Job drawing, mm, ordinate dimensions from the low corner. One solid piece. A direction names the side the tool comes from. Coordinates: 2 decimals unless noted, no trailing zeros. Write each loop counter-clockwise with the first axis right and the second up, starting at its lowest first coordinate (ties: lowest second). Pieces come first, ordered by that corner, then holes.
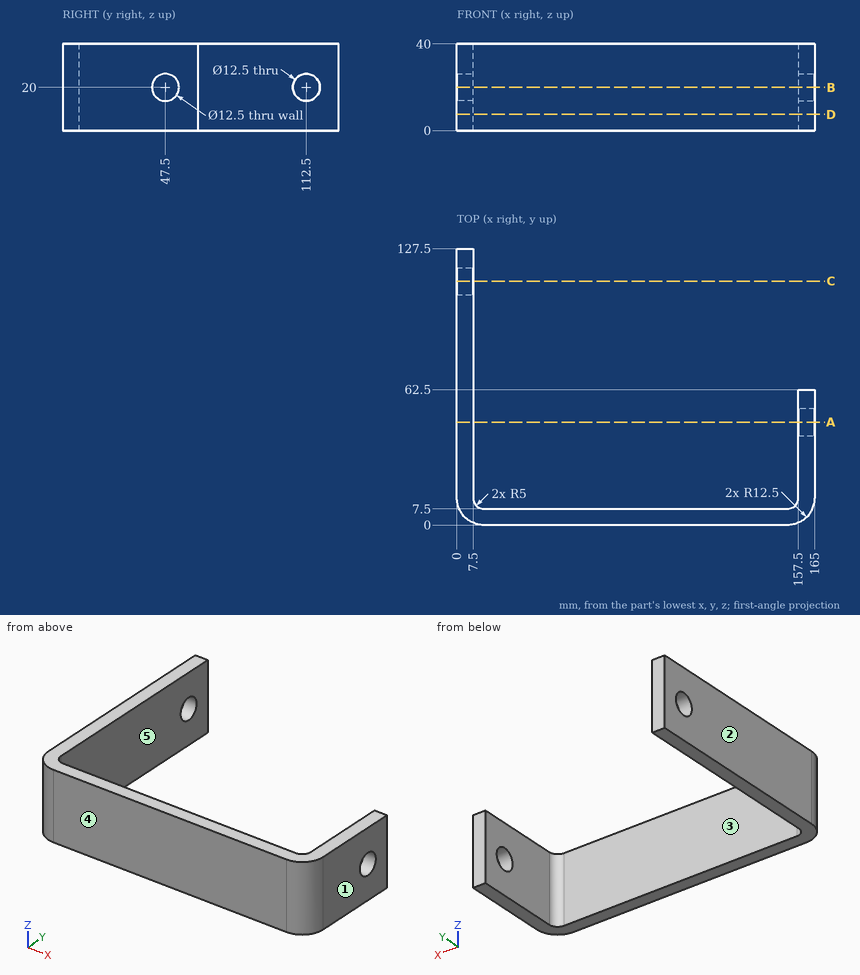
1. Flat gauge pins, fed straight in: pin 1 (1.5 mm diameter, centred on y = 82.5, z = 28.5, fed in from +X); pin 2 (6 mm diameter, centred on x = 161, z = 27.5, fed in from +Y); pin 3 (8 mm diameter, centred on x = 28.5, z = 23, fed in from +Y). Where does each tip first touch, or does it go through?
Computed values:
pin 1: stops at x = 7.5
pin 2: stops at y = 62.5
pin 3: stops at y = 7.5
2. Saw through at B-B on z = 20. List the corners of the cut face in (x, y).
Computed values:
outline: (0, 12.5) arc R12.5 ccw to (12.5, 0) - (152.5, 0) arc R12.5 ccw to (165, 12.5) - (165, 41.25) - (157.5, 41.25) - (157.5, 12.5) arc R5 cw to (152.5, 7.5) - (12.5, 7.5) arc R5 cw to (7.5, 12.5) - (7.5, 106.25) - (0, 106.25) - close; (0, 118.75) - (7.5, 118.75) - (7.5, 127.5) - (0, 127.5) - close; (157.5, 53.75) - (165, 53.75) - (165, 62.5) - (157.5, 62.5) - close
3. Saw through at A-A on y = 47.5. List the corners of the cut face in (x, z).
Computed values:
outline: (0, 0) - (7.5, 0) - (7.5, 40) - (0, 40) - close; (157.5, 0) - (165, 0) - (165, 13.75) - (157.5, 13.75) - close; (157.5, 26.25) - (165, 26.25) - (165, 40) - (157.5, 40) - close
4. Mould opens along X. For the marked faces 1, 2 and 3 say: +X half, -X half, draft (parallel to the pull), parting line (faces both ways), or undercut.
Computed values:
face 1: +X half
face 2: -X half
face 3: undercut
5. 3-axis set-ups, long thin cutter, end or side, ignore diameter. For the marked faces 4 and 5: which of +Z, -Z, +X, -X, +Y, -Y reach the whole face in a straight line?
Computed values:
face 4: +Z, -Z, +X, -X, -Y
face 5: +Z, -Z, +Y
6. Probe line 1 along X through (y, z) = (60.5, 30); line 2 along Z through (x, y) = (5, 112.5); line 3 along X through (y, z) = (82.5, 23.5). List the from-to ranges inside material, lowest first.
Computed values:
line 1: x = 0 to 7.5, 157.5 to 165
line 2: z = 0 to 13.75, 26.25 to 40
line 3: x = 0 to 7.5
7. Saw through at C-C on y = 112.5. List the corners of the cut face in (x, z).
Computed values:
outline: (0, 0) - (7.5, 0) - (7.5, 13.75) - (0, 13.75) - close; (0, 26.25) - (7.5, 26.25) - (7.5, 40) - (0, 40) - close
8. Saw through at D-D on z = 7.5. List the corners of the cut face in (x, y).
Computed values:
outline: (0, 12.5) arc R12.5 ccw to (12.5, 0) - (152.5, 0) arc R12.5 ccw to (165, 12.5) - (165, 62.5) - (157.5, 62.5) - (157.5, 12.5) arc R5 cw to (152.5, 7.5) - (12.5, 7.5) arc R5 cw to (7.5, 12.5) - (7.5, 127.5) - (0, 127.5) - close
